Check sheet for the modelled part. Datum: model origin and axes. Units: mm. A direction names the side the tool comes from. Give positions to 0.01 mm unless a question says otherwise; leave off trailing zeros. Loops run counter-clockwise (first coordinate to the right, second up) from the corner with the lowest first, then second, coordinate; pieces in that order, holes last. Notation, with made-up numbers: M -8.5,81 L 8.5,81 A14 ccw 8.5,88 Z; hole C 29,7 d7. An arc over 180 degrees is marked long. Write each question's results on one line, items separated by ' | '. Start each with the question number.
1. Material ranges on line 1 along X through (y, z) = (3, 0); line 2 along Y through (x, z) = (-3.75, 5); line 3 along X through (y, z) = (3.75, 0), recorded low to high.
2. Sectioned sample at B-B on z = 0. Give the number of separate pieces and of enclosed holes in the cut face, and give its area (3 significant figures).
3. Sectioned sample at C-C on x = 13.75. Record the cut outline in (y, z).
4. Tool access check on faces 1 (the flat face through (16.45, 3, 0)), 2 (the flat face through (13, 3, -3.5)), 3 (the flat face through (6.1, 4.5, -1.9)), 4 (the flat face through (12, 3, 3.5)), 5 (the flat face through (6, 7, 0)). Record the directions out of +Z, -Z, +X, -X, +Y, -Y that give a thin tool (end or side, any length) a straight path to the whole face; none if there is none.
5. Go/stop test with flat-tipped pins: pin 1 (7.5 mm diameter, centred on x = 0, z = 0, fed in from -Y); pin 2 (1 mm diameter, centred on x = -3.5, y = 5.5, fed in from +Z); pin 3 (3.5 mm diameter, centred on x = 14.5, y = 3.5, fed in from -Z). Record where each tip stops, or that it passes through.
6. Sectioned sample at A-A on y = 6.75. Record the cut outline in (x, z) (3 decimals), and give its area (3 significant figures).
7. Draft check along X on faces 6 (the flat face through (6, 0, 0)), 7 (the flat face through (5.019, 5.722, 4.477)), 8 (the flat face through (17.49, 3.45, 1.95)), 9 (the flat face through (6.1, 2.5, 1.9)). Enter one of: pulls with the +X half, pulls with the -X half, needs draft (parallel to the pull), parting line crosses it, or undercut.
```python
from build123d import *

# Parameters (mm, degrees)
SKETCH1_R           = 4.55
BOSS_EXTRUDE2_DEPTH = 7


with BuildPart() as part:
    # Sketch1 → Boss-Extrude2 (new body)
    with BuildSketch(Plane(origin=(0, 0, 0), x_dir=(1, 0, 0), z_dir=(0, 1, 0))):
        with BuildLine():
            Line((6.5, 3.5), (3.577981651, 5.426605505))
            ThreePointArc((3.577981651, 5.426605505), (-6.5, 0), (3.577981651, -5.426605505))
            Line((3.577981651, -5.426605505), (6.5, -3.5))
            Line((6.5, -3.5), (18.5, -3.5))
            Line((18.5, -3.5), (18.5, -1.655))
            Line((18.5, -1.655), (16.45, -2.255))
            Line((16.45, -2.255), (16.45, 2.255))
            Line((16.45, 2.255), (18.5, 1.655))
            Line((18.5, 1.655), (18.5, 3.5))
            Line((18.5, 3.5), (6.5, 3.5))
        make_face()
        with Locations(Location((0, 0, 0), (0, 0, 270))):
            Circle(SKETCH1_R, mode=Mode.SUBTRACT)
    extrude(amount=BOSS_EXTRUDE2_DEPTH)

    # Sketch2 → Cut-Revolve1 (revolve, cut)
    with BuildSketch(Plane(origin=(0, 0, 0), x_dir=(0, -1, 0), z_dir=(1, 0, 0))):
        with BuildLine():
            Line((-4.5, 6.805), (-4.5, 6.195))
            add(Edge.make_bspline(
                [(-4.5, 6.195), (-4.5, 5.595), (-3.5, 5.595), (-2.5, 5.595), (-2.5, 6.195)],
                knots=[0, 0, 0, 1.570796327, 1.570796327, 3.141592654, 3.141592654, 3.141592654], degree=2, weights=[1, 0.707106781, 1, 0.707106781, 1]))
            Line((-2.5, 6.195), (-2.5, 6.805))
            add(Edge.make_bspline(
                [(-2.5, 6.805), (-2.499999858, 7.405000085), (-3.5, 7.405000085), (-4.500000142, 7.405000085), (-4.5, 6.805)],
                knots=[3.141592512, 3.141592512, 3.141592512, 4.71238898, 4.71238898, 6.283185449, 6.283185449, 6.283185449], degree=2, weights=[1, 0.707106731, 1, 0.707106731, 1]))
        make_face()
    revolve(axis=Axis((0, 7.335318457, 0), (0, -1, 0)), mode=Mode.SUBTRACT)


solid = part.part
```
Output values:
1) line 1: -5.68 to -4.55, 4.55 to 5.68, 7.32 to 16.45 | line 2: 0 to 2.5, 4.5 to 7 | line 3: -5.61 to -4.55, 4.55 to 5.61, 7.39 to 16.45
2) separate pieces: 2 | enclosed holes: 1 | area: 92.3 mm2
3) outline: M 0,-3.5 L 7,-3.5 L 7,3.5 L 0,3.5 Z
4) face 1: +Y, -Y | face 2: -Z, +X, +Y, -Y | face 3: none | face 4: +Z, +X, +Y, -Y | face 5: +Z, -Z, +X, -X, +Y
5) pin 1: through | pin 2: z = 5.77 | pin 3: z = -3.5
6) outline: M 3.578,-5.427 L 6.5,-3.5 L 18.5,-3.5 L 18.5,-1.655 L 16.45,-2.255 L 16.45,2.255 L 18.5,1.655 L 18.5,3.5 L 6.5,3.5 L 3.578,5.427 A6.5 ccw long Z; hole C 0,0 d9.1 | area: 147 mm2
7) face 6: needs draft | face 7: pulls with the +X half | face 8: undercut | face 9: undercut
